from build123d import *

# Parameters (mm, degrees)
CUT_EXTRUDE1_DEPTH = 10
SWEEP1_PROFILE_R   = 0.3
SWEEP2_PROFILE_R   = 0.25


with BuildPart() as part:
    # Sketch1 → Revolve1 (revolve)
    with BuildSketch(Plane(origin=(0, 0, 0), x_dir=(0, 0, -1), z_dir=(1, 0, 0))):
        with BuildLine():
            Line((0, 0), (0, 8.6))
            ThreePointArc((0, 8.6), (1.732411614, 7.882411614), (2.45, 6.15))
            Line((2.45, 6.15), (2.45, 1))
            Line((2.45, 1), (2.9, 1))
            Line((2.9, 1), (2.9, 0))
            Line((2.9, 0), (0, 0))
        make_face()
    revolve(axis=Axis((0, 0, 0), (0, 1, 0)))

    # Sketch2 → Cut-Extrude1 (cut)
    with BuildSketch(Plane(origin=(0, 1, 0), x_dir=(1, 0, 0), z_dir=(0, 1, 0))):
        Polygon((0, 2.45), (-2.000825275, 2.45), (-0.041843052, 4.408982223), (3.123853817, 2.45), align=None)
    extrude(amount=-CUT_EXTRUDE1_DEPTH, mode=Mode.SUBTRACT)

    # Sweep1: sweep along a path in Sketch3
    with BuildLine(Plane(origin=(0, 0, 0), x_dir=(0, 0, -1), z_dir=(1, 0, 0))) as sweep1_path:
        Line((1.27, 0), (1.27, -18.255708098))
    # Sweep1 profile (on start of the path) → Sweep1 (sweep)
    with BuildSketch(Plane(origin=(0, 0, -1.27), x_dir=(0, 0, -1), z_dir=(0, -1, 0))):
        Circle(SWEEP1_PROFILE_R)
    sweep(path=sweep1_path.line)

    # Sweep2: sweep along a path in Sketch3<3>
    with BuildLine(Plane(origin=(0, 0, 0), x_dir=(0, 0, -1), z_dir=(1, 0, 0))) as sweep2_path:
        Line((-1.27, 0), (-1.27, -22))
    # Sweep2 profile (on start of the path) → Sweep2 (sweep)
    with BuildSketch(Plane(origin=(0, 0, 1.27), x_dir=(0, 0, -1), z_dir=(0, -1, 0))):
        Circle(SWEEP2_PROFILE_R)
    sweep(path=sweep2_path.line)


solid = part.part
Input: part model. Units: mm. Frame: model coordinates. A direction names the side the tool comes from. Round coordinates to 2 decimals unless told otherwise and drop trailing zeros. Order: outer loops, then holes, each group sorted by start corner. A loop starts at its lowest first (then second) coordinate and runs counter-clockwise, first axis right, second up. Notation, with made-up numbers: (-38.5, 58.25) - (-15.5, 58.25) arc R8 ccw to (-15.5, 72.25) - close; hole circle Ø5 at (32.5, 4.25). An arc over 180 degrees is marked (long way). Answer as a JSON object with one key per item and string values. Group by question number.
(1) Cut plane C-C (x = -1). Return loops of the section in (y, z).
(2) Cut plane D-D (z = -1.27). Return loops of the section in (x, y).
(3) Reachability of faces 1 (the face through (2.4, 3.5, 0.5)), 2 (the face through (-0.1, 0.5, 2.9)) from +Z, -Z, +X, -X, +Y, -Y: full face, straight path, thin tool, end or side. Return the list, or none.
(4) Cut plane B-B (z = 0). Return loops of the section in (x, y).
(5) Cut plane A-A (y = -13). Return loops of the section in (x, z), then the cut area to 3 significant figures.
(6) Pin query (flat end, axial travel): P1, Ø3, axis at y = 4, z = 1.5, coming from the -X side; P2, Ø3, axis at y = -2, z = 0.5, coming from the +X side; P3, Ø2, axis at x = 0, z = -1, coming from the +Y side; P4, Ø1, axis at x = 1.5, z = -2, coming from the -Y side. Return the tip coordinate at first contact, or that it passes through.
(7) Material intervals for probe 1 along Z at (x, y) = (-0.05, -14); probe 2 along Y at (x, z) = (0.8, 2.7); probe 3 along X at (y, z) = (-11, -1.35), sorted ascending. Write a range as from..to.
Here are the results:
{
 "1": {"outline": "(0, -2.45) - (1, -2.45) - (1, -2.24) - (6.15, -2.24) arc R2.24 ccw to (6.15, 2.24) - (1, 2.24) - (1, 2.72) - (0, 2.72) - close"},
 "2": {"outline": "(-2.61, 0) - (-0.3, 0) - (-0.3, -18.26) - (0.3, -18.26) - (0.3, 0) - (2.61, 0) - (2.61, 1) - (2.1, 1) - (2.1, 6.15) arc R2.1 ccw to (-2.1, 6.15) - (-2.1, 1) - (-2.61, 1) - close"},
 "3": {"face 1": "+Y", "face 2": "+Y, -Y"},
 "4": {"outline": "(-2.9, 0) - (2.9, 0) - (2.9, 1) - (2.45, 1) - (2.45, 6.15) arc R2.45 ccw to (-2.45, 6.15) - (-2.45, 1) - (-2.9, 1) - close"},
 "5": {"outline": "circle Ø0.6 at (0, -1.27); circle Ø0.5 at (0, 1.27)", "area": "0.479 mm^2"},
 "6": {"P1": "stops at x = -2.45", "P2": "stops at x = 0.25", "P3": "stops at y = 8.6", "P4": "stops at y = 0"},
 "7": {"probe 1": "z = -1.57..-0.97, 1.03..1.51", "probe 2": "y = 0..1", "probe 3": "x = -0.29..0.29"}
}
